Autodesk Inventor part; units mm, degrees
ref_plane "YZ Plane" through (0, 0, 0) normal (1, 0, 0) x (0, 1, 0)
ref_plane "XZ Plane" through (0, 0, 0) normal (0, 1, 0) x (-1, 0, 0)
ref_plane "XY Plane" through (0, 0, 0) normal (0, 0, 1) x (1, 0, 0)
sketch "Эскиз1" plane through (0, 0, 0) normal (0, 1, 0) x (-1, 0, 0)
  circle A0 centre (0, 0) radius 9.5
  circle A1 centre (0, 0) radius 3
  dimension "d0" = 19
  dimension "d1" = 6
extrude "Выдавливание1" add sketch "Эскиз1" along normal blind 6
sketch "Эскиз2" plane through (0, 6, 0) normal (0, 1, 0) x (1, 0, 0)
  circle A0 centre (0, 0) radius 4
  circle A1 centre (0, 0) radius 8.5
  circle A2 centre (0, 0) radius 9.5
  circle A3 centre (0, 0) radius 3
  dimension "d4" = 1
  dimension "d5" = 1
extrude "Выдавливание2" cut sketch "Эскиз2" against normal blind 0.5 contours A1
sketch "Эскиз3" plane through (0, 0, 0) normal (0, -1, 0) x (1, 0, 0)
  circle A0 centre (0, 0) radius 4
  circle A1 centre (0, 0) radius 8.5
extrude "Выдавливание3" cut sketch "Эскиз3" against normal blind 0.5
chamfer "Фаска1" distance 0.2 angle 45 8 edges at (-4, 0, 0) (3, 0, 0) (-8.5, 0, 0) (9.5, 0, 0) (9.5, 6, 0) (-8.5, 6, 0) (-4, 6, 0) (3, 6, 0)
properties part number "Подшипник 626Z" material "Титан"
Work out the finished part from the listing and answer in its coordinate system (mm). A direction names the side the tool comes from. Coordinates: 2 decimals unless noted, no trailing zeros. Loops run counter-clockwise (first coordinate to the right, second up) from the corner with the lowest first, then second, coordinate; pieces in that order, holes last. Notation, with made-up numbers: (78, 8.5) - (97, 8.5) arc R17 ccw to (97, 17.5) - close; hole circle Ø2 at (13.5, -6). An arc over 180 degrees is marked (long way). Use a Markdown table: item, result.
Item 1: Consider probe 1 along Z at (x, y) = (0, 5.75); probe 2 along X at (y, z) = (5.7, -3.5); probe 3 along Y at (x, z) = (4, 6.5). Determine where each line is inside the solid, lowest interval first. Write a range as from..to.
Evaluation:
| item | result |
|---|---|
| probe 1 | z = -9.5..-8.5, -4..-3, 3..4, 8.5..9.5 |
| probe 2 | x = -8.83..-7.75, -1.94..1.94, 7.75..8.83 |
| probe 3 | y = 0.5..5.5 |
Item 2: Find section A-A, the plane y = 3.75. Determine the outline of the cut face in (x, z).
Evaluation:
| item | result |
|---|---|
| outline | circle Ø19 at (0, 0); hole circle Ø6 at (0, 0) |
Item 3: For faces 1 (the cylindrical face through (8.11, 0.35, 2.55)), 2 (the flat face through (2, 6, -3)), 3 (the cylindrical face through (8.11, 5.65, -2.55)), determine the directions among +Z, -Z, +X, -X, +Y, -Y from which every point of the face is accessible in a straight line to the end or side of a thin tool.
Evaluation:
| item | result |
|---|---|
| face 1 | -Y |
| face 2 | +Z, -Z, +X, -X, +Y |
| face 3 | +Y |
Item 4: Given pin 1 Ø2 at (x, z) = (4.5, 2.5) entering from -Y; pin 2 Ø5 at (x, z) = (0, 0) entering from +Y; pin 3 Ø2 at (x, y) = (-5, 1.5) entering from +Z; pin 4 Ø2 at (x, y) = (-3, 2) entering from -Z, each flat-ended and moving along its own axis, determine where each tip first touches the part or whether it passes through.
Evaluation:
| item | result |
|---|---|
| pin 1 | stops at y = 0.5 |
| pin 2 | passes through |
| pin 3 | stops at z = 8.62 |
| pin 4 | stops at z = -9.29 |
Item 5: The mould has two halves that part along X. Classify faces 4 (the cylindrical face through (3, 3, 0)), 5 (the flat face through (2, 0, -3)): +X half, -X half, draft (parallel to the pull), parting line (faces both ways), or undercut.
Evaluation:
| item | result |
|---|---|
| face 4 | undercut |
| face 5 | draft |
